CAD build for the part. Positions are in the model's coordinates, mm. A direction names the side the tool comes from. Give positions to 0.01 mm unless a question says otherwise; leave off trailing zeros. Order: outer loops, then holes, each group sorted by start corner. A loop starts at its lowest first (then second) coordinate and runs counter-clockwise, first axis right, second up. Notation, with made-up numbers: M -16,-38.75 L 21,-38.75 A18 cw 21,-3.75 Z; hole C 46.25,6 d3. An arc over 180 degrees is marked long. Put each result on its own line as item: value. Start each with the question number.
1) Drill centre lines: line 1 (X direction, y = 0.15, z = 0); line 2 (Y direction, x = -3, z = 3.25); line 3 (X direction, y = 1.8, z = -0.5). Where is each one in solid material? Low to high. Write a range as [from, to].
2) Cut at D-D (x = -4). Write the cut outline in (y, z), and give its area (3 significant figures).
3) Tool access for faces 1 (the face through (-2.44, 1.48, -0.54)), 2 (the face through (3, 2.9, 0)): list every direction of +Z, -Z, +X, -X, +Y, -Y with a clear straight run to the whole face (end or side of a thin tool).
4) Pin check, flat tip, straight feed: pin 1 (1.5 mm diameter, centred on y = 2.5, z = -1.5, fed in from -X). Stop position of the tip, or through.
5) Two-plate mould, pull along X, no slides. Class faces 3 (the face through (-4.88, 1.48, -1.08)), 4 (the face through (-3, 0.1, 0)): released by +X, released by -X, zero draft, split by the parting line, or undercut.
6) Cut at C-C (y = 2.7). Write the cut outline in (x, z), and give its area (3 significant figures).
7) Cut at A-A (z = 0). Write the cut outline in (x, y).
8) Cut at B-B (x = 0). Write the cut outline in (y, z).
```python
from build123d import *

# Parameters (mm, degrees)
SKETCH1_R           = 5
SKETCH1_R_2         = 2.5
BOSS_EXTRUDE1_DEPTH = 3
SKETCH2_R           = 4.725189579
SKETCH2_R_2         = 2.787282072
CUT_EXTRUDE1_DEPTH  = 0.1
CUT_EXTRUDE2_START  = -0.1
SKETCH3_R           = 4.725189579
SKETCH3_R_2         = 2.787282072
CUT_EXTRUDE2_DEPTH  = 0.1


with BuildPart() as part:
    # Sketch1 → Boss-Extrude1 (new body)
    with BuildSketch(Plane(origin=(0, 0, 0), x_dir=(1, 0, 0), z_dir=(0, 1, 0))):
        with Locations(Location((0, 0, 0), (0, 0, 270))):
            Circle(SKETCH1_R)
        with Locations(Location((0, 0, 0), (0, 0, 270))):
            Circle(SKETCH1_R_2, mode=Mode.SUBTRACT)
    extrude(amount=BOSS_EXTRUDE1_DEPTH)

    # Sketch2 → Cut-Extrude1 (cut)
    with BuildSketch(Plane.XZ):
        with Locations(Location((0, 0, 0), (0, 0, 270))):
            Circle(SKETCH2_R)
        with Locations(Location((0, 0, 0), (0, 0, 270))):
            Circle(SKETCH2_R_2, mode=Mode.SUBTRACT)
    extrude(amount=-CUT_EXTRUDE1_DEPTH, mode=Mode.SUBTRACT)

    # Sketch3 → Cut-Extrude2 (cut)
    with BuildSketch(Plane(origin=(0, 3, 0), x_dir=(1, 0, 0), z_dir=(0, 1, 0)).offset(CUT_EXTRUDE2_START)):
        with Locations(Location((0, 0, 0), (0, 0, 90))):
            Circle(SKETCH3_R)
        with Locations(Location((0, 0, 0), (0, 0, 90))):
            Circle(SKETCH3_R_2, mode=Mode.SUBTRACT)
    extrude(amount=CUT_EXTRUDE2_DEPTH, mode=Mode.SUBTRACT)


solid = part.part
```
Solution:
1. line 1: [-5, -2.5], [2.5, 5]
1. line 2: [0.1, 2.9]
1. line 3: [-4.97, -2.45], [2.45, 4.97]
2. outline: M 0,-3 L 3,-3 L 3,-2.52 L 2.9,-2.52 L 2.9,2.52 L 3,2.52 L 3,3 L 0,3 L 0,2.52 L 0.1,2.52 L 0.1,-2.52 L 0,-2.52 Z
2. area: 17.0 mm²
3. face 1: +Y, -Y
3. face 2: +Y
4. pin 1: x = -4.94
5. face 3: split by the parting line
5. face 4: undercut
6. outline: C 0,0 d10; hole C 0,0 d5
6. area: 58.9 mm²
7. outline: M -5,0 L -4.73,0 L -4.73,0.1 L -2.79,0.1 L -2.79,0 L -2.5,0 L -2.5,3 L -2.79,3 L -2.79,2.9 L -4.73,2.9 L -4.73,3 L -5,3 Z; M 2.5,0 L 2.79,0 L 2.79,0.1 L 4.73,0.1 L 4.73,0 L 5,0 L 5,3 L 4.73,3 L 4.73,2.9 L 2.79,2.9 L 2.79,3 L 2.5,3 Z
8. outline: M 0,-5 L 3,-5 L 3,-4.73 L 2.9,-4.73 L 2.9,-2.79 L 3,-2.79 L 3,-2.5 L 0,-2.5 L 0,-2.79 L 0.1,-2.79 L 0.1,-4.73 L 0,-4.73 Z; M 0,2.5 L 3,2.5 L 3,2.79 L 2.9,2.79 L 2.9,4.73 L 3,4.73 L 3,5 L 0,5 L 0,4.73 L 0.1,4.73 L 0.1,2.79 L 0,2.79 Z
